from build123d import *

# Parameters (mm, degrees)
F0_W     = 1.2
F0_H     = 33
F1_DEPTH = 30


with BuildPart() as f1:
    # F0 (on Front) → F1 (new body)
    with BuildSketch(Plane.XZ):
        with Locations((0.6, 16.5)):
            Rectangle(F0_W, F0_H)
        with BuildLine():
            ThreePointArc((-7, 40), (-2.050253, 37.949747), (0, 33))
            Line((0, 33), (1.2, 33))
            ThreePointArc((1.2, 33), (-1.201724, 38.798276), (-7, 41.2))
            Line((-7, 41.2), (-12, 41.2))
            Line((-12, 41.2), (-12, 40))
            Line((-12, 40), (-7, 40))
        make_face()
    extrude(amount=F1_DEPTH)


solid = f1.part
Geometry: final body of the model. Coordinates: model frame, mm. A direction names the side the tool comes from. Give positions to 0.01 mm unless a question says otherwise; leave off trailing zeros. Loops run counter-clockwise (first coordinate to the right, second up) from the corner with the lowest first, then second, coordinate; pieces in that order, holes last. Notation, with made-up numbers: M -21.5,42 L 16.5,42 A21 ccw 16.5,72 Z; hole C 59.5,-0.75 d2. An arc over 180 degrees is marked long. Put each result on its own line as item: value. Start each with the question number.
1) Cut plane B-B (z = 20). Output: boundary loops of the cut face in (x, y).
2) Contact query for flat-ended pins moving along their axis: pin 1 (6 mm diameter, centred on y = -4.5, z = 16, fed in from -X); pin 2 (4 mm diameter, centred on x = -8.5, y = -10, fed in from -Z); pin 3 (3 mm diameter, centred on x = -0.5, y = -16, fed in from +Z). Output: stop coordinate, or through.
3) Ray query, line 1 along Z through (x, y) = (-10, -24.5); line 2 along X through (y, z) = (-8.25, 9); line 3 along X through (y, z) = (-1.25, 39). Return the intervals inside material, ascending.
4) Cut plane A-A (y = -19.5). Output: boundary loops of the cut face in (x, z).
5) Access query for faces 1 (the flat face through (-10, -15, 40)), 2 (the cylindrical face through (-1.138, -14.79, 38.734)). Directions: +Z, -Z, +X, -X, +Y, -Y. A direction counts if a zero-diameter tool reaches every point of the face in a straight line with its end or side. Return the directions, or none.
6) Cut plane C-C (x = -8). Output: boundary loops of the cut face in (y, z).
Verdict:
1. outline: M 0,-30 L 1.2,-30 L 1.2,0 L 0,0 Z
2. pin 1: x = 0
2. pin 2: z = 39.98
2. pin 3: z = 39.5
3. line 1: 40 to 41.2
3. line 2: 0 to 1.2
3. line 3: -3.39 to -1.41
4. outline: M -12,40 L -7,40 A7 cw 0,33 L 0,0 L 1.2,0 L 1.2,33 A8.2 ccw -7,41.2 L -12,41.2 Z
5. face 1: -Z, -X, +Y, -Y
5. face 2: +Z, +X, +Y, -Y
6. outline: M -30,40 L 0,40 L 0,41.2 L -30,41.2 Z
